Solid Edge part; units mm, degrees
sketch "Sketch1" plane through (0, 0, 0) normal (0, 0, 1) x (1, 0, 0)
  line L0 (11.50209, -20) -> (11.50209, 0)
  line L1 (11.50209, 0) -> (3.884116, 30.955848)
  line L2 (3.50209, -20) -> (-3.955194, 29.402971)
  line L3 (3.50209, -20) -> (11.50209, -20)
  arc A0 (-3.955198, 29.403) -> (3.884126, 30.955806) centre (0, 30) cw
  circle A1 centre (5.001393, 10) radius 1.5
  circle A2 centre (0, 30) radius 1.5
extrude "Protrusion1" add sketch "Sketch1" along normal blind 12
sketch "Sketch2" plane through (3.751045, 7, 12) normal (0, 0, 1) x (0, -1, 0)
  line L0 (27, 3.751045) -> (27, 7.751045)
  line L1 (27, 7.751045) -> (7, 7.751045)
  line L2 (7, 7.751045) -> (7, 3.751045)
  line L3 (7, 3.751045) -> (27, 3.751045)
extrude "Cutout1" cut sketch "Sketch2" against normal through all
sketch "Sketch3" plane through (0, 0, 0) normal (1, 0, 0) x (0, 1, 0)
  line L0 (1.5, 10) -> (34, 10)
  line L1 (34, 10) -> (34, 2)
  line L2 (34, 2) -> (1.5, 2)
  line L3 (1.5, 2) -> (1.5, 10)
extrude "Cutout2" cut sketch "Sketch3" along normal through all and the other way through all
fillet "Redondeo_1" radius 5 1 edges at (0.256706, 1.5, 6)
fillet "Redondeo_2" radius 3 1 edges at (3.50209, -20, 6)
chamfer "Chaflán_1" distance 0.5 angle 45 25 edges at (-0.419179, 5.9776, 12) (-0.777251, 33.923758, 12) (7.693103, 15.477924, 12) (11.50209, 0, 6) (7.693103, 15.477924, 0) (-0.777251, 33.923758, 0) (-0.419179, 5.9776, 0) (4.126616, -19.274128, 12) (6.792661, -20, 12) (4.126616, -19.274128, 0) (6.792661, -20, 0) (-1.415548, 12.578343, 10) (-0.777251, 33.923758, 10) (7.508534, 16.227924, 10) (11.132952, 1.5, 6) (7.508534, 16.227924, 2) (-1.415548, 12.578343, 2) (0, 28.5, 2) (5.001393, 8.5, 2) (3.501393, 10, 12) (-1.5, 30, 12) (-1.5, 30, 0) (3.501393, 10, 0) (3.501393, 10, 10) (7.50209, -20, 6)
Read the model definition and answer for the solid it produces. Units are mm, in the model's axes. A direction names the side the tool comes from. Give positions to 0.01 mm unless a question says otherwise; leave off trailing zeros. Write each loop counter-clockwise with the first axis right and the second up, starting at its lowest first coordinate (ties: lowest second). Pieces come first, ordered by that corner, then holes. Notation, with made-up numbers: (63.25, 57.25) - (78.25, 57.25) arc R23 cw to (78.25, 68.25) - close; hole circle Ø1 at (16.5, 29.25). An arc over 180 degrees is marked (long way). Answer in a Markdown table with one row per item. Add a question column.
Item 1: Section A-A, the plane y = 30 is taken. Count the separate pieces of the cut face and the enclosed holes in it, and give its area (3 significant figures).
Item 2: Determine the mould class of faces 4 (the face through (-0.784, 33.557, 11.858)), 5 (the face through (4.34, -18.986, 0.142)), 6 (the face through (9, 0, 6)), 7 (the face through (-0.784, 33.557, 1.858)) for opening direction Z: pulls with the +Z half, pulls with the -Z half, needs draft (parallel to the pull), parting line crosses it, or undercut.
Item 3: Find the intervals of material crossed by L1, parallel to Z at x = 3.25, y = 9; L2, parallel to Z at x = 0.75, y = -0.5; L3, parallel to X at y = 30, z = 10.95, in increasing order.
Item 4: A tool of negligible diameter and unlimited length cuts with its end or side. For faces 1 (the face through (7.271, 16.134, 10.247)), 2 (the face through (7.502, -10, 6)), 3 (the face through (4, 7, 12)), from which of +Z, -Z, +X, -X, +Y, -Y can it reach the whole face along a straight path? Write none if from no direction.
Item 5: Section C-C, the plane z = 5.5 is taken. Write down the section's boundary in (x, y).
Item 6: Flat-ended cylindrical pins translate along their axes: P1, Ø2.5, axis at x = 8, z = 7, coming from the +Y side; P2, Ø6, axis at y = -14.5, z = 5.5, coming from the +X side; P3, Ø2, axis at x = 6.5, y = 5, coming from the -Z side; P4, Ø1.5, axis at x = 8.5, z = 8, coming from the -Y side. Find the tip coordinate at first contact, or state that the pin passes through.
Recorded:
| question | item | result |
|---|---|---|
| 1 | separate pieces | 4 |
| 1 | enclosed holes | 0 |
| 1 | area | 18.7 mm2 |
| 2 | face 4 | pulls with the +Z half |
| 2 | face 5 | pulls with the -Z half |
| 2 | face 6 | needs draft |
| 2 | face 7 | undercut |
| 3 | L1 | z = 0 to 2, 10 to 12 |
| 3 | L2 | z = 0.31 to 1.69, 10.31 to 11.69 |
| 3 | L3 | x = -4 to -1.5, 1.5 to 4.12 |
| 4 | face 1 | +X, +Y |
| 4 | face 2 | +Z, -Z, +X, -Y |
| 4 | face 3 | +Z, +X, -X, +Y, -Y |
| 5 | outline | (1.12, -4.25) - (3.12, -17.45) arc R3 ccw to (6.08, -20) - (7, -20) - (7.5, -19.5) - (7.5, 0) - (11, 0) - (11.38, 0.49) - (11.25, 1.01) - (10.63, 1.5) - (6.07, 1.5) arc R5 ccw to start |
| 6 | P1 | stops at y = 1.5 |
| 6 | P2 | stops at x = 7.5 |
| 6 | P3 | stops at z = 0 |
| 6 | P4 | stops at y = 0 |
